from build123d import *

# Parameters (mm, degrees)
EXTRUDE_1_DEPTH = 140


with BuildPart() as part:
    # ｽｹｯﾁ1 → ﾎﾞｽ - 押し出し1 (new body)
    with BuildSketch(Plane.XY):
        with BuildLine():
            Line((-40, -77), (-25, -43.301270189))
            ThreePointArc((-25, -43.301270189), (0, -50), (25, -43.301270189))
            Line((25, -43.301270189), (40, -77))
            Line((40, -77), (40, -80))
            Line((40, -80), (80, -80))
            Line((80, -80), (80, -67))
            Line((80, -67), (46.494717001, -67))
            Line((46.494717001, -67), (33.281076638, -37.314473571))
            ThreePointArc((33.281076638, -37.314473571), (0, 50), (-33.281076638, -37.314473571))
            Line((-33.281076638, -37.314473571), (-46.494717001, -67))
            Line((-46.494717001, -67), (-80, -67))
            Line((-80, -67), (-80, -80))
            Line((-80, -80), (-40, -80))
            Line((-40, -80), (-40, -77))
        make_face()
    extrude(amount=EXTRUDE_1_DEPTH)


solid = part.part
Can you work these out from the model? Positions are in its coordinate system, mm. A direction names the side the tool comes from. Give positions to 0.01 mm unless a question says otherwise; leave off trailing zeros. Order: outer loops, then holes, each group sorted by start corner. A loop starts at its lowest first (then second) coordinate and runs counter-clockwise, first axis right, second up. Notation, with made-up numbers: M 27,83 L 43,83 A29 ccw 43,111 Z; hole C -18,-25.75 d4. An arc over 180 degrees is marked long. Use a Markdown table: item, result. Add a question column.
Item 1: For faces 1 (the flat face through (39.98, -52.365, 69.02)), 2 (the flat face through (-1, -14, 0)), 3 (the flat face through (-32.605, -60.387, 69.02)), 4 (the flat face through (-39.795, -51.949, 69.02)), which set-ups out of +Z, -Z, +X, -X, +Y, -Y let a thin tool reach every point of the face, with its end or its side?
Item 2: Suppose I cut it at A-A (z = 48.5). List the corners of the cut face in (x, y) for me, then the cut area to 3 significant figures.
Item 3: If I drill on L1, parallel to Y at x = -72.5, z = 15; L2, parallel to X at y = -62.5, z = 124; L3, parallel to X at y = -63, z = 101, over which ranges is the centre line in solid material (lowest first)? Write a range as [from, to].
Item 4: Will these pins go through, and if not, where does the flat tip stop? pin 1 (1.5 mm diameter, centred on y = -42.5, z = 23, fed in from -X); pin 2 (5 mm diameter, centred on x = -46, z = 78.5, fed in from +Y); pin 3 (2 mm diameter, centred on y = -50, z = 62, fed in from -X).
Item 5: Suppose I cut it at B-B (x = 0). List the corners of the cut face in (y, z) for me.
Item 6: We'd pull the mould along X, two halves only. Please class faces 5 (the cylindrical face through (1.69, 49.97, 69.02)), 6 (the flat face through (32.395, -59.915, 69.02)), 7 (the flat face through (80, -74, 69)): +X half, -X half, draft (parallel to the pull), parting line (faces both ways), or undercut.
Answer sheet:
| question | item | result |
|---|---|---|
| 1 | face 1 | +Z, -Z, +X |
| 1 | face 2 | -Z, +X, -X, +Y, -Y |
| 1 | face 3 | +Z, -Z, -Y |
| 1 | face 4 | +Z, -Z, -X |
| 2 | outline | M -80,-80 L -40,-80 L -40,-77 L -25,-43.3 A50 ccw 25,-43.3 L 40,-77 L 40,-80 L 80,-80 L 80,-67 L 46.49,-67 L 33.28,-37.31 A50 ccw long -33.28,-37.31 L -46.49,-67 L -80,-67 Z |
| 2 | area | 9,520 mm² |
| 3 | L1 | y = [-80, -67] |
| 3 | L2 | x = [-44.49, -33.55], [33.55, 44.49] |
| 3 | L3 | x = [-44.71, -33.77], [33.77, 44.71] |
| 4 | pin 1 | stops at x = -35.92 |
| 4 | pin 2 | stops at y = 24.65 |
| 4 | pin 3 | stops at x = -39.37 |
| 5 | outline | M -50,0 L 50,0 L 50,140 L -50,140 Z |
| 6 | face 5 | parting line |
| 6 | face 6 | undercut |
| 6 | face 7 | +X half |
